Input: part model. Units: mm. Frame: model coordinates. Face numbers are marked on the shaded views. A direction names the side the tool comes from. Coordinates: 2 decimals unless noted, no trailing zeros. Loops run counter-clockwise (first coordinate to the right, second up) from the corner with the lowest first, then second, coordinate; pieces in that order, holes last. Notation, with made-up numbers: (86, 21.5) -> (94, 21.5) arc R11 ccw to (94, 29.5) -> close; hole circle Ø3 at (7.5, -25.75). An arc over 180 degrees is marked (long way). Put each result on its own line as item: value. Start each with the question number.
1) Cut plane B-B (z = 4). Return the cut outline in (x, y), plus the area to 3 significant figures.
2) Cut plane D-D (z = -15.5). Return the cut outline in (x, y), plus the area to 3 significant figures.
3) Set-up query: the marked faces 1, 2 and 3. Return all of +Z, -Z, +X, -X, +Y, -Y with unobstructed straight access to the full face (end or side cutting, diameter ignored); none if empty.
4) Pull-direction query (Y, two-part tool) for the marked faces 4, 5 and 6; classes: pulls with the +Y half, pulls with the -Y half, needs draft (parallel to the pull), parting line crosses it, or undercut.
5) Cut plane A-A (y = -25.5). Return the cut outline in (x, z).
6) Contact query for flat-ended pins moving along their axis: P1, Ø3.5, axis at x = -15.5, z = -16, coming from the +Y side; P2, Ø1.3, axis at y = 11.5, z = -1, coming from the -X side; P3, Ø12, axis at x = 1, z = -9.5, coming from the +Y side; P4, Ø0.6, axis at x = 18, z = -20.5, coming from the -Y side. Output: stop coordinate, or through.
7) Cut plane C-C (x = -15.5). Return the cut outline in (y, z).
8) Material intervals for L1, parallel to Z at x = 15.5, y = -7.25; L2, parallel to X at y = -4, z = -15, sorted ascending.
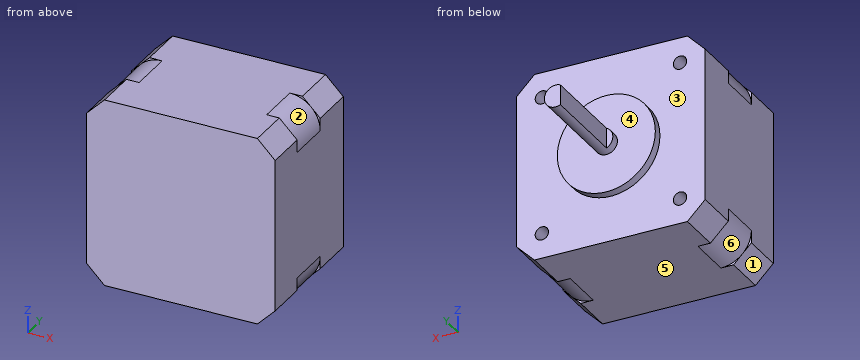
from build123d import *

# Parameters (mm, degrees)
F0_W      = 42.3
F0_H      = 42.3
F1_DEPTH  = 29.5
F2_R      = 11
F3_DEPTH  = 2
F4_R      = 2.5
F5_DEPTH  = 22
F7_DEPTH  = 20
F8_SIZE   = 4
F11_DEPTH = 5
F12_R     = 1.5
F13_DEPTH = 10


with BuildPart() as f1:
    # F0 (on Front) → F1 (new body)
    with BuildSketch(Plane.XZ):
        Rectangle(F0_W, F0_H)
    extrude(amount=F1_DEPTH)

    # F2 (on face) → F3 (join)
    with BuildSketch(Plane(origin=(0, 0, 0), x_dir=(-1, 0, 0), z_dir=(0, 1, 0))):
        Circle(F2_R)
    extrude(amount=F3_DEPTH)

    # F4 (on face) → F5 (join)
    with BuildSketch(Plane(origin=(0, 2, 0), x_dir=(-1, 0, 0), z_dir=(0, 1, 0))):
        Circle(F4_R)
    extrude(amount=F5_DEPTH)

    # F6 (on face) → F7 (cut)
    with BuildSketch(Plane(origin=(0, 24, 0), x_dir=(-1, 0, 0), z_dir=(0, 1, 0))):
        with BuildLine():
            ThreePointArc((2.5, 0), (2.1182908015, 1.3277213865), (1.0897247359, 2.25))
            Line((1.0897247359, 2.25), (1.0897247359, -2.25))
            ThreePointArc((1.0897247359, -2.25), (2.1182908015, -1.3277213865), (2.5, 0))
        make_face()
    extrude(amount=-F7_DEPTH, mode=Mode.SUBTRACT)

    # F8
    f8_edges = [f1.edges().sort_by_distance(p)[0] for p in [
        (-21.15, -14.75, 21.15),
        (-21.15, -14.75, -21.15),
        (21.15, -14.75, -21.15),
        (21.15, -14.75, 21.15),
    ]]
    chamfer(f8_edges, length=F8_SIZE)

    # F10 (on offset) → F11 (cut, symmetric)
    with BuildSketch(Plane.XZ.offset(15)):
        with BuildLine():
            ThreePointArc((14.3215728753, 21.15), (19.15, 19.15), (21.15, 14.3215728753))
            Line((21.15, 14.3215728753), (21.15, 21.15))
            Line((21.15, 21.15), (14.3215728753, 21.15))
        make_face()
        with BuildLine():
            Line((-21.15, 21.15), (-21.15, 14.3215728753))
            ThreePointArc((-21.15, 14.3215728753), (-19.15, 19.15), (-14.3215728753, 21.15))
            Line((-14.3215728753, 21.15), (-21.15, 21.15))
        make_face()
        with BuildLine():
            Line((21.15, -21.15), (21.15, -14.3215728753))
            ThreePointArc((21.15, -14.3215728753), (19.15, -19.15), (14.3215728753, -21.15))
            Line((14.3215728753, -21.15), (21.15, -21.15))
        make_face()
        with BuildLine():
            ThreePointArc((-14.3215728753, -21.15), (-19.15, -19.15), (-21.15, -14.3215728753))
            Line((-21.15, -14.3215728753), (-21.15, -21.15))
            Line((-21.15, -21.15), (-14.3215728753, -21.15))
        make_face()
    extrude(amount=F11_DEPTH, both=True, mode=Mode.SUBTRACT)

    # F12 (on face) → F13 (cut)
    with BuildSketch(Plane(origin=(0, 0, 0), x_dir=(-1, 0, 0), z_dir=(0, 1, 0))):
        with Locations((-15.5, 15.5)):
            Circle(F12_R)
        with Locations((15.5, 15.5)):
            Circle(F12_R)
        with Locations((-15.5, -15.5)):
            Circle(F12_R)
        with Locations((15.5, -15.5)):
            Circle(F12_R)
    extrude(amount=-F13_DEPTH, mode=Mode.SUBTRACT)


solid = f1.part
Results found:
1. outline: (-21.15, -29.5) -> (21.15, -29.5) -> (21.15, 0) -> (10.25, 0) -> (10.25, 2) -> (-10.25, 2) -> (-10.25, 0) -> (-21.15, 0) -> close
1. area: 1,290 mm2
2. outline: (-21.15, -29.5) -> (21.15, -29.5) -> (21.15, -20) -> (21.05, -20) -> (21.05, -10) -> (21.15, -10) -> (21.15, 0) -> (17, 0) -> (17, -10) -> (14, -10) -> (14, 0) -> (-14, 0) -> (-14, -10) -> (-17, -10) -> (-17, 0) -> (-21.15, 0) -> (-21.15, -10) -> (-21.05, -10) -> (-21.05, -20) -> (-21.15, -20) -> close
2. area: 1,190 mm2
3. face 1: -Z, -X, +Y, -Y
3. face 2: +Z, +X
3. face 3: +Y
4. face 4: pulls with the +Y half
4. face 5: needs draft
4. face 6: undercut
5. outline: (-21.15, -17.15) -> (-17.15, -21.15) -> (17.15, -21.15) -> (21.15, -17.15) -> (21.15, 17.15) -> (17.15, 21.15) -> (-17.15, 21.15) -> (-21.15, 17.15) -> close
6. P1: stops at y = 0
6. P2: stops at x = -1.09
6. P3: stops at y = 2
6. P4: stops at y = -29.5
7. outline: (-29.5, -21.15) -> (-20, -21.15) -> (-20, -21.05) -> (-10, -21.05) -> (-10, -21.15) -> (0, -21.15) -> (0, -17) -> (-10, -17) -> (-10, -14) -> (0, -14) -> (0, 14) -> (-10, 14) -> (-10, 17) -> (0, 17) -> (0, 21.15) -> (-10, 21.15) -> (-10, 21.05) -> (-20, 21.05) -> (-20, 21.15) -> (-29.5, 21.15) -> close
8. L1: z = -21.15 to -17, -14 to 14, 17 to 21.15
8. L2: x = -21.15 to -16.91, -14.09 to 14.09, 16.91 to 21.15
